Check sheet for the modelled part. Datum: model origin and axes. Units: mm. A direction names the side the tool comes from. Round coordinates to 2 decimals unless told otherwise and drop trailing zeros. Loops run counter-clockwise (first coordinate to the right, second up) from the corner with the lowest first, then second, coordinate; pieces in that order, holes last. Notation, with made-up numbers: (74, 1.5) - (130, 1.5) arc R19 cw to (130, 21.5) - close; hole circle Ø6 at (39.25, 25.25). An arc over 180 degrees is marked (long way). Return JSON: item names as keys, results as strings.
from build123d import *
from OCP.BRepFilletAPI import BRepFilletAPI_MakeChamfer

# Parameters (mm, degrees)
SKETCH1_W                 = 241
SKETCH1_H                 = 12.7
BOSS_EXTRUDE1_DEPTH       = 25.4
CHAMFER1_SIZE             = 8
CHAMFER1_SIZE2            = 50
M5X0_8_TAPPED_HOLE1_D     = 4.2
M5X0_8_TAPPED_HOLE1_DEPTH = 12
M5X0_8_TAPPED_HOLE1_TIP   = 1.2618073
FILLET1_R                 = 10


with BuildPart() as part:
    # Sketch1 → Boss-Extrude1 (new body)
    with BuildSketch(Plane(origin=(0, 0, 0), x_dir=(1, 0, 0), z_dir=(0, 1, 0))):
        Rectangle(SKETCH1_W, SKETCH1_H)
    extrude(amount=BOSS_EXTRUDE1_DEPTH)

    # Chamfer1: one chamfer whose edges measure the first distance from different faces: ONE call of the kernel's chamfer builder (chamfer() names one face for all edges)
    chamfer1_edges_1 = [part.edges().sort_by_distance(p)[0] for p in [
        (-120.5, 25.4, 0),
    ]]
    chamfer1_side_1 = [part.faces().sort_by_distance(p)[0] for p in [
        (-120.5, 12.7, 0),
    ]]
    chamfer1_edges_2 = [part.edges().sort_by_distance(p)[0] for p in [
        (120.5, 25.4, 0),
    ]]
    chamfer1_side_2 = [part.faces().sort_by_distance(p)[0] for p in [
        (120.5, 12.7, 0),
    ]]
    chamfer1 = BRepFilletAPI_MakeChamfer(part.part.solid().wrapped)
    for e in chamfer1_edges_1:
        chamfer1.Add(CHAMFER1_SIZE, CHAMFER1_SIZE2, e.wrapped, chamfer1_side_1[0].wrapped)  # the first distance lies on this face
    for e in chamfer1_edges_2:
        chamfer1.Add(CHAMFER1_SIZE, CHAMFER1_SIZE2, e.wrapped, chamfer1_side_2[0].wrapped)  # the first distance lies on this face
    add(Compound.cast(chamfer1.Shape()), mode=Mode.REPLACE)

    # M5x0.8 Tapped Hole1
    with Locations(Plane(origin=(0, 0, 0), x_dir=(-1, 0, 0), z_dir=(0, -1, 0))):
        with Locations((112.5, 0), (67.5, 0), (22.5, 0), (-22.5, 0), (-67.5, 0), (-112.5, 0)):
            Hole(M5X0_8_TAPPED_HOLE1_D / 2, depth=M5X0_8_TAPPED_HOLE1_DEPTH)
            with Locations((0, 0, -(M5X0_8_TAPPED_HOLE1_DEPTH + M5X0_8_TAPPED_HOLE1_TIP / 2))):  # 118° drill point
                Cone(0, M5X0_8_TAPPED_HOLE1_D / 2, M5X0_8_TAPPED_HOLE1_TIP, mode=Mode.SUBTRACT)

    # Fillet1
    fillet1_edges = [part.edges().sort_by_distance(p)[0] for p in [
        (-70.5, 25.4, 0),
        (70.5, 25.4, 0),
        (120.5, 17.4, 0),
        (-120.5, 17.4, 0),
    ]]
    fillet(fillet1_edges, radius=FILLET1_R)


solid = part.part
Q1. Scan lines: probe 1 along Z at (x, y) = (-112.5, 5.5); probe 2 along Y at (x, z) = (84, -4.75); probe 3 along X at (y, z) = (17.5, 5.5). Record each from-to range of solid material in increasing order. Write a range as [from, to].
Answer key:
{"probe 1": "z = [-6.35, -2.1], [2.1, 6.35]", "probe 2": "y = [0, 23.24]", "probe 3": "x = [-115.56, 115.56]"}
Q2. Tool access check on faces 4 (the face through (69.44, 6.08, 0.8)), 5 (the face through (120.5, 4, 0)). Record the directions out of +Z, -Z, +X, -X, +Y, -Y that give a thin tool (end or side, any length) a straight path to the whole face; none if there is none.
Answer key:
{"face 4": "-Y", "face 5": "+Z, -Z, +X, +Y, -Y"}
Q3. Depth check by flat-ended pin: P1, Ø3, axis at y = 18.5, z = 2.5, coming from the +X side; P2, Ø4, axis at y = 17, z = 2.5, coming from the -X side; P3, Ø5, axis at x = -112.5, z = 0, coming from the +Y side. Enter the tip coordinate at first touch or a pass-through.
Answer key:
{"P1": "stops at x = 116.33", "P2": "stops at x = -118.4", "P3": "stops at y = 19.08"}
Q4. Sectioned sample at B-B (y = 3.75). Enter the section's corners in (x, z).
Answer key:
{"outline": "(-120.5, -6.35) - (120.5, -6.35) - (120.5, 6.35) - (-120.5, 6.35) - close; hole circle Ø4.2 at (-112.5, 0); hole circle Ø4.2 at (-67.5, 0); hole circle Ø4.2 at (-22.5, 0); hole circle Ø4.2 at (22.5, 0); hole circle Ø4.2 at (67.5, 0); hole circle Ø4.2 at (112.5, 0)"}
Q5. Draft check along X on faces 1 (the face through (-2, 13, 6.35)), 2 (the face through (118.17, 15.29, -0.09)), 3 (the face through (-112.84, 13.04, 0.14)). Enter one of: released by +X, released by -X, zero draft, split by the parting line, or undercut.
Answer key:
{"face 1": "zero draft", "face 2": "released by +X", "face 3": "undercut"}
Q6. Sectioned sample at A-A (z = 4.25). Enter the section's corners in (x, y), plus the area to 3 significant figures.
Answer key:
{"outline": "(-120.5, 0) - (120.5, 0) - (120.5, 8.87) arc R10 ccw to (112.08, 18.75) - (71.28, 25.27) arc R10 ccw to (69.71, 25.4) - (-69.71, 25.4) arc R10 ccw to (-71.28, 25.27) - (-112.08, 18.75) arc R10 ccw to (-120.5, 8.87) - close", "area": "5,690 mm²"}
Q7. Sectioned sample at C-C (y = 22.5). Enter the section's corners in (x, z) (3 decimals).
Answer key:
{"outline": "(-88.625, -6.35) - (88.625, -6.35) - (88.625, 6.35) - (-88.625, 6.35) - close"}
